from build123d import *

# Parameters (mm, degrees)
F0_W     = 5
F0_H     = 5
F0_R     = 6
F1_DEPTH = 440


with BuildPart() as f1:
    # F0 (on Front) → F1 (new body)
    with BuildSketch(Plane.XZ):
        with BuildLine():
            Line((5, -20), (18, -20))
            ThreePointArc((18, -20), (19.414214, -19.414214), (20, -18))
            Line((20, -18), (20, -5))
            Line((20, -5), (16, -5))
            Line((16, -5), (16, -11.5))
            Line((16, -11.5), (12.914214, -11.5))
            Line((12.914214, -11.5), (9, -7.585786))
            Line((9, -7.585786), (9, 0))
            Line((9, 0), (9, 7.585786))
            Line((9, 7.585786), (12.914214, 11.5))
            Line((12.914214, 11.5), (16, 11.5))
            Line((16, 11.5), (16, 5))
            Line((16, 5), (20, 5))
            Line((20, 5), (20, 18))
            ThreePointArc((20, 18), (19.414214, 19.414214), (18, 20))
            Line((18, 20), (5, 20))
            Line((5, 20), (5, 16))
            Line((5, 16), (11.5, 16))
            Line((11.5, 16), (11.5, 12.914214))
            Line((11.5, 12.914214), (7.585786, 9))
            Line((7.585786, 9), (0, 9))
            Line((0, 9), (-7.585786, 9))
            Line((-7.585786, 9), (-11.5, 12.914214))
            Line((-11.5, 12.914214), (-11.5, 16))
            Line((-11.5, 16), (-5, 16))
            Line((-5, 16), (-5, 20))
            Line((-5, 20), (-18, 20))
            ThreePointArc((-18, 20), (-19.414214, 19.414214), (-20, 18))
            Line((-20, 18), (-20, 5))
            Line((-20, 5), (-16, 5))
            Line((-16, 5), (-16, 11.5))
            Line((-16, 11.5), (-12.914214, 11.5))
            Line((-12.914214, 11.5), (-9, 7.585786))
            Line((-9, 7.585786), (-9, 0))
            Line((-9, 0), (-9, -7.585786))
            Line((-9, -7.585786), (-12.914214, -11.5))
            Line((-12.914214, -11.5), (-16, -11.5))
            Line((-16, -11.5), (-16, -5))
            Line((-16, -5), (-20, -5))
            Line((-20, -5), (-20, -18))
            ThreePointArc((-20, -18), (-19.414214, -19.414214), (-18, -20))
            Line((-18, -20), (-5, -20))
            Line((-5, -20), (-5, -16))
            Line((-5, -16), (-11.5, -16))
            Line((-11.5, -16), (-11.5, -12.914214))
            Line((-11.5, -12.914214), (-7.585786, -9))
            Line((-7.585786, -9), (0, -9))
            Line((0, -9), (7.585786, -9))
            Line((7.585786, -9), (11.5, -12.914214))
            Line((11.5, -12.914214), (11.5, -16))
            Line((11.5, -16), (5, -16))
            Line((5, -16), (5, -20))
        make_face()
        with Locations((-16, -16)):
            Rectangle(F0_W, F0_H, mode=Mode.SUBTRACT)
        with Locations((16, -16)):
            Rectangle(F0_W, F0_H, mode=Mode.SUBTRACT)
        with Locations((-16, 16)):
            Rectangle(F0_W, F0_H, mode=Mode.SUBTRACT)
        Circle(F0_R, mode=Mode.SUBTRACT)
        with Locations((16, 16)):
            Rectangle(F0_W, F0_H, mode=Mode.SUBTRACT)
    extrude(amount=F1_DEPTH)


solid = f1.part
Build history of the part. All positions in model axes, mm. A direction names the side the tool comes from. Round coordinates to 2 decimals unless told otherwise and drop trailing zeros. Order: outer loops, then holes, each group sorted by start corner. A loop starts at its lowest first (then second) coordinate and runs counter-clockwise, first axis right, second up. Notation, with made-up numbers: M 26.5,30.5 L 72.5,30.5 A31 ccw 72.5,60.5 Z; hole C 86.25,-16.5 d9. An arc over 180 degrees is marked long. Use CSV: the item, a comma, the result in double quotes. Start each with the question number.
(1) Tool access for faces 1 (the face through (-20, -217, -11)), 2 (the face through (-9, -217, 0)): list every direction of +Z, -Z, +X, -X, +Y, -Y with a clear straight run to the whole face (end or side of a thin tool).
(2) Cut at A-A on z = 0. List the corners of the cut face in (x, y).
(3) Cut at B-B on x = 0. List the corners of the cut face in (y, z), then the cut area to 3 significant figures.
(4) Cut at C-C on y = -213. State how many separate pieces and enclosed holes the cut face has, then the cut area to 3 significant figures.
(5) Flat gauge pin, fed straight in: P1, Ø6, axis at y = -286.5, z = 1, coming from the -X side. Where does the tip first touch, or does it go through?
(6) Drill centre lines: probe 1 along X at (y, z) = (-287.5, 15); probe 2 along Z at (x, y) = (7.5, -403); probe 3 along X at (y, z) = (-203.5, 17.5). Where is each one in solid material? Low to high.
(7) Mould opens along Z. For faces 3 (the face through (-11, -217, 20)), 4 (the face through (11, -217, -20)), 5 (the face through (-5, -440, -4)), 6 (the face through (0, -217, 9)) say: +Z half, -Z half, draft (parallel to the pull), parting line (faces both ways), or undercut.
Findings:
1,face 1,"+Z, -Z, -X, +Y, -Y"
1,face 2,"+Y, -Y"
2,outline,"M -9,-440 L -6,-440 L -6,0 L -9,0 Z; M 6,-440 L 9,-440 L 9,0 L 6,0 Z"
3,outline,"M -440,-9 L 0,-9 L 0,-6 L -440,-6 Z; M -440,6 L 0,6 L 0,9 L -440,9 Z"
3,area,"2,640 mm^2"
4,separate pieces,"1"
4,enclosed holes,"5"
4,area,"641 mm^2"
5,P1,"stops at x = -9"
6,probe 1,"x = -20 to -18.5, -13.5 to -11.5, 11.5 to 13.5, 18.5 to 20"
6,probe 2,"z = -20 to -16, -9 to 9, 16 to 20"
6,probe 3,"x = -20 to -18.5, -13.5 to -5, 5 to 13.5, 18.5 to 20"
7,face 3,"+Z half"
7,face 4,"-Z half"
7,face 5,"draft"
7,face 6,"undercut"
